Model file for the job. Use its own axes, mm. Face numbers are marked on the shaded views. A direction names the side the tool comes from. Coordinates: 2 decimals unless noted, no trailing zeros. Write each loop counter-clockwise with the first axis right and the second up, starting at its lowest first coordinate (ties: lowest second). Pieces come first, ordered by that corner, then holes. Notation, with made-up numbers: (71.25, -35.5) - (120.25, -35.5) arc R13 cw to (120.25, -28.5) - close; hole circle Ø6 at (-20.75, -11.75). An arc over 180 degrees is marked (long way). Put each result on its own line as item: value. Start each with the question number.
1. Saw through at C-C, the plane z = 19. Write the cut outline in (x, y), plus the area to 3 significant figures.
2. Pull direction Y, two halves, no side cores. Call the marked faces 1, 2 and 3: released by +Y, released by -Y, zero draft, split by the parting line, or undercut.
3. Drill centre lines: L1, parallel to Z at x = -2, y = 5; L2, parallel to Y at x = 0.5, z = 32; L3, parallel to Z at x = -5, y = 0.5. Where is each one in solid material? Low to high. Write a range as from..to.
4. Drop flat-ended pins along their axis: P1, Ø2, axis at y = 2, z = 19.5, coming from the -X side; P2, Ø5, axis at y = -5.5, z = 17.5, coming from the -X side; P3, Ø4, axis at x = 0, y = 0, coming from the -Z side; P4, Ø5, axis at x = 1.5, z = 4, coming from the -Y side. Give the stop position or say it passes through.
5. Which spindle directions (+Z, -Z, +X, -X, +Y, -Y) get a long thin tool onto all of the face, cutting with end or side? Do the marked faces 4, 5 and 6. Say none if no direction does.
6. Saw through at D-D, the plane z = 7. Write the cut outline in (x, y), plus the area to 3 significant figures.
7. Saw through at A-A, the plane y = 0. Write the cut outline in (x, z), plus the area to 3 significant figures.
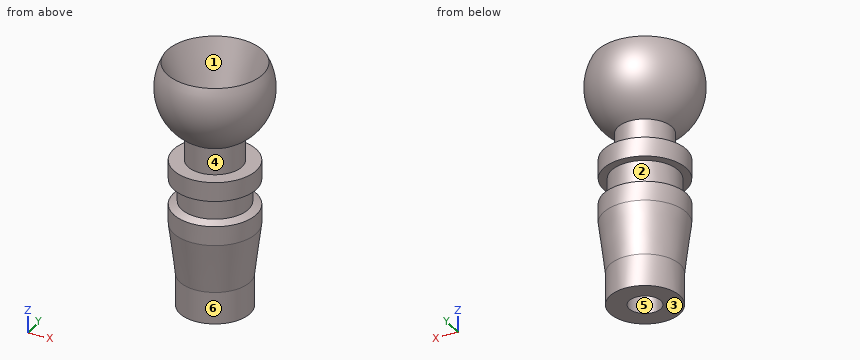
```python
from build123d import *


with BuildPart() as part:
    # Sketch3 → Revolve1 (revolve)
    with BuildSketch(Plane(origin=(0, 0, 0), x_dir=(1, 0, 0), z_dir=(0, 1, 0)), mode=Mode.PRIVATE) as revolve1_sk:
        with BuildLine():
            Line((2.5, 0), (5.5, 0))
            Line((5.5, 0), (5.5, -5))
            Line((5.5, -5), (6.5, -13))
            Line((6.5, -13), (6.5, -16))
            Line((6.5, -16), (5.25, -16.5))
            Line((5.25, -16.5), (5.25, -20))
            Line((5.25, -20), (6.5, -20))
            Line((6.5, -20), (6.5, -23))
            Line((6.5, -23), (4.25, -23))
            Line((4.25, -23), (4.25, -26))
            Line((4.25, -26), (4.25, -27.138784068))
            ThreePointArc((4.25, -27.138784068), (8.172615224, -32.16368658), (7.498594715, -38.502633796))
            Line((7.498594715, -38.502633796), (2.5, -27.138784068))
            Line((2.5, -27.138784068), (2.5, 0))
        make_face()
    revolve(revolve1_sk.sketch.rotate(Axis((0, 0, -88.99), (0, 0, 1)), 180), axis=Axis((0, 0, -88.99), (0, 0, 1)))


solid = part.part
```
Final values:
1. outline: circle Ø10.5 at (0, 0); hole circle Ø5 at (0, 0)
1. area: 67.0 mm²
2. face 1: undercut
2. face 2: split by the parting line
2. face 3: zero draft
3. L1: z = 0..16.45, 20..23, 27.92..33.7
3. L2: y = -8.11..-4.61, 4.61..8.11
3. L3: z = 0..23, 27.64..32.88
4. P1: stops at x = -6.4
4. P2: stops at x = -5.48
4. P3: passes through
4. P4: stops at y = -5.64
5. face 4: none
5. face 5: +Z, -Z
5. face 6: -Z
6. outline: circle Ø11.5 at (0, 0); hole circle Ø5 at (0, 0)
6. area: 84.2 mm²
7. outline: (-7.5, 38.5) arc R8.5 ccw to (-4.25, 27.14) - (-4.25, 23) - (-6.5, 23) - (-6.5, 20) - (-5.25, 20) - (-5.25, 16.5) - (-6.5, 16) - (-6.5, 13) - (-5.5, 5) - (-5.5, 0) - (-2.5, 0) - (-2.5, 27.14) - close; (2.5, 0) - (5.5, 0) - (5.5, 5) - (6.5, 13) - (6.5, 16) - (5.25, 16.5) - (5.25, 20) - (6.5, 20) - (6.5, 23) - (4.25, 23) - (4.25, 27.14) arc R8.5 ccw to (7.5, 38.5) - (2.5, 27.14) - close
7. area: 230 mm²
